from build123d import *

# Parameters (mm, degrees)
F0_W      = 60
F0_H      = 60
F0_R      = 22.4096796893
F1_DEPTH  = 3
F2_W      = 60
F2_H      = 60
F2_W_2    = 54
F2_H_2    = 54
F3_DEPTH  = 15
F4_W      = 135
F4_H      = 75
F4_W_2    = 54
F4_H_2    = 54
F5_DEPTH  = 3
F6_W      = 135
F6_H      = 75
F6_W_2    = 129
F6_H_2    = 69
F7_DEPTH  = 25
F8_W      = 195
F8_H      = 75
F8_W_2    = 129
F8_H_2    = 69
F9_DEPTH  = 3
F10_W     = 15
F10_H     = 68
F11_DEPTH = 25
F12_W     = 15
F12_H     = 75
F13_DEPTH = 25
F15_DEPTH = 200
F17_DEPTH = 25
F18_R     = 3.49999
F21_DEPTH = 60


# Not quite as in the source:
# - a fillet or chamfer is up to 0.001 mm smaller than in the source, because OpenCascade refuses the exact size


with BuildPart() as f1:
    # F0 (on Front) → F1 (new body)
    with BuildSketch(Plane.XZ):
        Rectangle(F0_W, F0_H)
        Circle(F0_R, mode=Mode.SUBTRACT)
    extrude(amount=F1_DEPTH)

    # F2 (on face) → F3 (join)
    with BuildSketch(Plane(origin=(0, 0, 0), x_dir=(-1, 0, 0), z_dir=(0, 1, 0))):
        Rectangle(F2_W, F2_H)
        Rectangle(F2_W_2, F2_H_2, mode=Mode.SUBTRACT)
    extrude(amount=F3_DEPTH)

    # F4 (on face) → F5 (join)
    with BuildSketch(Plane(origin=(0, 15, 0), x_dir=(-1, 0, 0), z_dir=(0, 1, 0))):
        Rectangle(F4_W, F4_H)
        Rectangle(F4_W_2, F4_H_2, mode=Mode.SUBTRACT)
    extrude(amount=F5_DEPTH)

    # F6 (on face) → F7 (join)
    with BuildSketch(Plane(origin=(0, 18, 0), x_dir=(-1, 0, 0), z_dir=(0, 1, 0))):
        Rectangle(F6_W, F6_H)
        Rectangle(F6_W_2, F6_H_2, mode=Mode.SUBTRACT)
    extrude(amount=F7_DEPTH)

    # F8 (on face) → F9 (join)
    with BuildSketch(Plane(origin=(0, 43, 0), x_dir=(-1, 0, 0), z_dir=(0, 1, 0))):
        Rectangle(F8_W, F8_H)
        Rectangle(F8_W_2, F8_H_2, mode=Mode.SUBTRACT)
    extrude(amount=F9_DEPTH)

    # F10 (on face) → F11 (join)
    with BuildSketch(Plane.XZ.offset(-43)):
        with Locations((-90, -3.5)):
            Rectangle(F10_W, F10_H)
    extrude(amount=F11_DEPTH)

    # F12 (on face) → F13 (join)
    with BuildSketch(Plane.XZ.offset(-43)):
        with Locations((90, 0)):
            Rectangle(F12_W, F12_H)
    extrude(amount=F13_DEPTH)

    # F14 (on face) → F15 (cut)
    with BuildSketch(Plane.XY.offset(37.5)):
        with BuildLine():
            ThreePointArc((-82.5, 27), (-90, 21.7838821814), (-97.5, 27))
            Line((-97.5, 27), (-97.5, 18))
            Line((-97.5, 18), (-82.5, 18))
            Line((-82.5, 18), (-82.5, 27))
        make_face()
        with BuildLine():
            ThreePointArc((97.5, 27), (90, 21.7838821814), (82.5, 27))
            Line((82.5, 27), (82.5, 18))
            Line((82.5, 18), (97.5, 18))
            Line((97.5, 18), (97.5, 27))
        make_face()
    extrude(amount=-F15_DEPTH, mode=Mode.SUBTRACT)

    # F16 (on face) → F17 (cut)
    with BuildSketch(Plane.XZ.offset(-43)):
        Polygon((-77.5, 37.5), (-82.5, 37.5), (-97.5, 37.5), (-97.5, 30.5), (-82.5, 30.5), (-77.5, 30.5), align=None)
    extrude(amount=-F17_DEPTH, mode=Mode.SUBTRACT)

    # F18 (radius 3.5 in the source; OpenCascade refuses exactly that, so slightly less here)
    f18_edges = [f1.edges().sort_by_distance(p)[0] for p in [
        (-77.5, 44.5, 30.5),
        (-77.5, 44.5, 37.5),
    ]]
    fillet(f18_edges, radius=F18_R)

    # F20 (on face) → F21 (cut)
    with BuildSketch(Plane.XY.offset(30)):
        Polygon((-30, -3), (-50, 15), (-50, -3), align=None)
    extrude(amount=-F21_DEPTH, mode=Mode.SUBTRACT)


solid = f1.part
Input: part model. Units: mm. Frame: model coordinates. A direction names the side the tool comes from. Give positions to 0.01 mm unless a question says otherwise; leave off trailing zeros. Loops run counter-clockwise (first coordinate to the right, second up) from the corner with the lowest first, then second, coordinate; pieces in that order, holes last. Notation, with made-up numbers: M 19,-28.5 L 76,-28.5 A28 ccw 76,-1.5 Z; hole C 1.25,-20.75 d2. An arc over 180 degrees is marked long. Use CSV: the item, a comma, the result in double quotes.
(1) Material intervals for L1, parallel to X at y = 36, z = -23.5; L2, parallel to X at y = 20, z = -7.5; L3, parallel to Z at x = -41.5, y = 21, sorted ascending. Write a range as [from, to].
Outcome:
L1,"x = [-97.5, -82.5], [-67.5, -64.5], [64.5, 67.5], [82.5, 97.5]"
L2,"x = [-67.5, -64.5], [64.5, 67.5]"
L3,"z = [-37.5, -34.5], [34.5, 37.5]"
(2) Section A-A, the plane z = 0. Return loops of the section in (x, y), plus the area to 3 significant figures.
Outcome:
outline,"M -97.5,27 A8 ccw -82.5,27 L -82.5,43 L -67.5,43 L -67.5,15 L -30,15 L -30,-3 L -22.41,-3 L -22.41,0 L -27,0 L -27,18 L -64.5,18 L -64.5,46 L -97.5,46 Z; M 22.41,-3 L 30,-3 L 30,15 L 67.5,15 L 67.5,43 L 82.5,43 L 82.5,27 A8 ccw 97.5,27 L 97.5,46 L 64.5,46 L 64.5,18 L 27,18 L 27,0 L 22.41,0 Z"
area,"1,320 mm²"
(3) Section D-D, the plane z = -24.5. Return loops of the section in (x, y), plus the area to 3 significant figures.
Outcome:
outline,"M -97.5,27 A8 ccw -82.5,27 L -82.5,43 L -67.5,43 L -67.5,15 L -30,15 L -30,-3 L 30,-3 L 30,15 L 67.5,15 L 67.5,43 L 82.5,43 L 82.5,27 A8 ccw 97.5,27 L 97.5,46 L 64.5,46 L 64.5,18 L 27,18 L 27,0 L -27,0 L -27,18 L -64.5,18 L -64.5,46 L -97.5,46 Z"
area,"1,450 mm²"
(4) Section C-C, the plane y = 2.5. Return loops of the section in (x, z).
Outcome:
outline,"M -30,-30 L 30,-30 L 30,30 L -30,30 Z; hole M -27,-27 L 27,-27 L 27,27 L -27,27 Z"
(5) Section B-B, the plane x = 0. Return loops of the section in (y, z), plus the area to 3 significant figures.
Outcome:
outline,"M -3,-30 L 15,-30 L 15,-37.5 L 46,-37.5 L 46,-34.5 L 18,-34.5 L 18,-27 L 0,-27 L 0,-22.41 L -3,-22.41 Z; M -3,22.41 L 0,22.41 L 0,27 L 18,27 L 18,34.5 L 46,34.5 L 46,37.5 L 15,37.5 L 15,30 L -3,30 Z"
area,"367 mm²"
(6) Set-up query: faces 1 (the face through (30, 18, 0)), 2 (the face through (82.5, 35, -1)), 3 (the face through (0, 6, 30)), 4 (the face through (-30, 6, 0)). Return all of +Z, -Z, +X, -X, +Y, -Y with unobstructed straight access to the full face (end or side cutting, diameter ignored); none if empty.
Outcome:
face 1,"+Y"
face 2,"+Z, -Z, -Y"
face 3,"+Z, +X, -X, -Y"
face 4,"+Z, -Z, -X, -Y"
(7) Pull-direction query (Z, two-part tool) for faces 5 (the face through (64.5, 32, 0)), 6 (the face through (0, 9, 27)), 7 (the face through (-67.5, 29, -1)), 8 (the face through (-89, 34, 30.5)); classes: pulls with the +Z half, pulls with the -Z half, needs draft (parallel to the pull), parting line crosses it, or undercut.
Outcome:
face 5,"undercut"
face 6,"undercut"
face 7,"needs draft"
face 8,"pulls with the +Z half"
(8) Pin query (flat end, axial travel): P1, Ø9, axis at x = 6.5, y = 12, coming from the +Z side; P2, Ø1, axis at x = -43, z = -24.5, coming from the -Y side; P3, Ø14.5, axis at x = 8, y = 2, coming from the +Z side; P4, Ø12, axis at x = 74, z = -3, coming from the -Y side. Return the tip coordinate at first contact, or that it passes through.
Outcome:
P1,"stops at z = 37.5"
P2,"stops at y = 15"
P3,"stops at z = 30"
P4,"stops at y = 43"
